```python
from build123d import *

# Parameters (mm, degrees)
SKETCH1_R           = 57.5
SKETCH1_R_2         = 1.75
SKETCH1_R_3         = 26
SKETCH1_R_4         = 2.5
BOSS_EXTRUDE1_DEPTH = 7
SKETCH2_R           = 7
SKETCH2_R_2         = 5
CUT_EXTRUDE1_DEPTH  = 1


with BuildPart() as part:
    # Sketch1 → Boss-Extrude1 (new body)
    with BuildSketch(Plane(origin=(0, 0, 0), x_dir=(1, 0, 0), z_dir=(0, 1, 0))):
        with Locations(Location((0, 0, 0), (0, 0, 270))):
            Circle(SKETCH1_R)
        with Locations(Location((0, 54, 0), (0, 0, 270))):
            Circle(SKETCH1_R_2, mode=Mode.SUBTRACT)
        with Locations(Location((27, 46.765371804, 0), (0, 0, 270))):
            Circle(SKETCH1_R_2, mode=Mode.SUBTRACT)
        with Locations(Location((46.765371804, 27, 0), (0, 0, 270))):
            Circle(SKETCH1_R_2, mode=Mode.SUBTRACT)
        with Locations(Location((54, 0, 0), (0, 0, 270))):
            Circle(SKETCH1_R_2, mode=Mode.SUBTRACT)
        with Locations(Location((46.765371804, -27, 0), (0, 0, 270))):
            Circle(SKETCH1_R_2, mode=Mode.SUBTRACT)
        with Locations(Location((27, -46.765371804, 0), (0, 0, 270))):
            Circle(SKETCH1_R_2, mode=Mode.SUBTRACT)
        with Locations(Location((0, -54, 0), (0, 0, 270))):
            Circle(SKETCH1_R_2, mode=Mode.SUBTRACT)
        with Locations(Location((-27, -46.765371804, 0), (0, 0, 270))):
            Circle(SKETCH1_R_2, mode=Mode.SUBTRACT)
        with Locations(Location((-46.765371804, -27, 0), (0, 0, 270))):
            Circle(SKETCH1_R_2, mode=Mode.SUBTRACT)
        with Locations(Location((-54, 0, 0), (0, 0, 270))):
            Circle(SKETCH1_R_2, mode=Mode.SUBTRACT)
        with Locations(Location((-46.765371804, 27, 0), (0, 0, 270))):
            Circle(SKETCH1_R_2, mode=Mode.SUBTRACT)
        with Locations(Location((-27, 46.765371804, 0), (0, 0, 270))):
            Circle(SKETCH1_R_2, mode=Mode.SUBTRACT)
        with Locations(Location((0, 0, 0), (0, 0, 270))):
            Circle(SKETCH1_R_3, mode=Mode.SUBTRACT)
        with Locations(Location((0, 45, 0), (0, 0, 270))):
            Circle(SKETCH1_R_4, mode=Mode.SUBTRACT)
        with Locations(Location((24.328836786, 37.856408977, 0), (0, 0, 270))):
            Circle(SKETCH1_R_4, mode=Mode.SUBTRACT)
        with Locations(Location((40.933439791, 18.693675585, 0), (0, 0, 270))):
            Circle(SKETCH1_R_4, mode=Mode.SUBTRACT)
        with Locations(Location((44.541964885, -6.404167722, 0), (0, 0, 270))):
            Circle(SKETCH1_R_4, mode=Mode.SUBTRACT)
        with Locations(Location((34.008730846, -29.468733028, 0), (0, 0, 270))):
            Circle(SKETCH1_R_4, mode=Mode.SUBTRACT)
        with Locations(Location((12.677965058, -43.177183813, 0), (0, 0, 270))):
            Circle(SKETCH1_R_4, mode=Mode.SUBTRACT)
        with Locations(Location((-12.677965058, -43.177183813, 0), (0, 0, 270))):
            Circle(SKETCH1_R_4, mode=Mode.SUBTRACT)
        with Locations(Location((-34.008730846, -29.468733028, 0), (0, 0, 270))):
            Circle(SKETCH1_R_4, mode=Mode.SUBTRACT)
        with Locations(Location((-44.541964885, -6.404167722, 0), (0, 0, 270))):
            Circle(SKETCH1_R_4, mode=Mode.SUBTRACT)
        with Locations(Location((-40.933439791, 18.693675585, 0), (0, 0, 270))):
            Circle(SKETCH1_R_4, mode=Mode.SUBTRACT)
        with Locations(Location((-24.328836786, 37.856408977, 0), (0, 0, 270))):
            Circle(SKETCH1_R_4, mode=Mode.SUBTRACT)
    extrude(amount=BOSS_EXTRUDE1_DEPTH)

    # Sketch2 → Cut-Extrude1 (cut)
    # profile 1 of 11: a face of its own
    with BuildSketch(Plane(origin=(0, 7, 0), x_dir=(1, 0, 0), z_dir=(0, 1, 0))):
        with Locations(Location((0, 45, 0), (0, 0, 270))):
            Circle(SKETCH2_R)
        with Locations(Location((0, 45, 0), (0, 0, 270))):
            Circle(SKETCH2_R_2, mode=Mode.SUBTRACT)
    # profile 2 of 11: a face of its own
    with BuildSketch(Plane(origin=(0, 7, 0), x_dir=(1, 0, 0), z_dir=(0, 1, 0))):
        with Locations(Location((24.328836786, 37.856408977, 0), (0, 0, 270))):
            Circle(SKETCH2_R)
        with Locations(Location((24.328836786, 37.856408977, 0), (0, 0, 270))):
            Circle(SKETCH2_R_2, mode=Mode.SUBTRACT)
    # profile 3 of 11: a face of its own
    with BuildSketch(Plane(origin=(0, 7, 0), x_dir=(1, 0, 0), z_dir=(0, 1, 0))):
        with Locations(Location((40.933439791, 18.693675585, 0), (0, 0, 270))):
            Circle(SKETCH2_R)
        with Locations(Location((40.933439791, 18.693675585, 0), (0, 0, 270))):
            Circle(SKETCH2_R_2, mode=Mode.SUBTRACT)
    # profile 4 of 11: a face of its own
    with BuildSketch(Plane(origin=(0, 7, 0), x_dir=(1, 0, 0), z_dir=(0, 1, 0))):
        with Locations(Location((44.541964885, -6.404167722, 0), (0, 0, 270))):
            Circle(SKETCH2_R)
        with Locations(Location((44.541964885, -6.404167722, 0), (0, 0, 270))):
            Circle(SKETCH2_R_2, mode=Mode.SUBTRACT)
    # profile 5 of 11: a face of its own
    with BuildSketch(Plane(origin=(0, 7, 0), x_dir=(1, 0, 0), z_dir=(0, 1, 0))):
        with Locations(Location((34.008730846, -29.468733028, 0), (0, 0, 270))):
            Circle(SKETCH2_R)
        with Locations(Location((34.008730846, -29.468733028, 0), (0, 0, 270))):
            Circle(SKETCH2_R_2, mode=Mode.SUBTRACT)
    # profile 6 of 11: a face of its own
    with BuildSketch(Plane(origin=(0, 7, 0), x_dir=(1, 0, 0), z_dir=(0, 1, 0))):
        with Locations(Location((12.677965058, -43.177183813, 0), (0, 0, 270))):
            Circle(SKETCH2_R)
        with Locations(Location((12.677965058, -43.177183813, 0), (0, 0, 270))):
            Circle(SKETCH2_R_2, mode=Mode.SUBTRACT)
    # profile 7 of 11: a face of its own
    with BuildSketch(Plane(origin=(0, 7, 0), x_dir=(1, 0, 0), z_dir=(0, 1, 0))):
        with Locations(Location((-12.677965058, -43.177183813, 0), (0, 0, 270))):
            Circle(SKETCH2_R)
        with Locations(Location((-12.677965058, -43.177183813, 0), (0, 0, 270))):
            Circle(SKETCH2_R_2, mode=Mode.SUBTRACT)
    # profile 8 of 11: a face of its own
    with BuildSketch(Plane(origin=(0, 7, 0), x_dir=(1, 0, 0), z_dir=(0, 1, 0))):
        with Locations(Location((-34.008730846, -29.468733028, 0), (0, 0, 270))):
            Circle(SKETCH2_R)
        with Locations(Location((-34.008730846, -29.468733028, 0), (0, 0, 270))):
            Circle(SKETCH2_R_2, mode=Mode.SUBTRACT)
    # profile 9 of 11: a face of its own
    with BuildSketch(Plane(origin=(0, 7, 0), x_dir=(1, 0, 0), z_dir=(0, 1, 0))):
        with Locations(Location((-44.541964885, -6.404167722, 0), (0, 0, 270))):
            Circle(SKETCH2_R)
        with Locations(Location((-44.541964885, -6.404167722, 0), (0, 0, 270))):
            Circle(SKETCH2_R_2, mode=Mode.SUBTRACT)
    # profile 10 of 11: a face of its own
    with BuildSketch(Plane(origin=(0, 7, 0), x_dir=(1, 0, 0), z_dir=(0, 1, 0))):
        with Locations(Location((-40.933439791, 18.693675585, 0), (0, 0, 270))):
            Circle(SKETCH2_R)
        with Locations(Location((-40.933439791, 18.693675585, 0), (0, 0, 270))):
            Circle(SKETCH2_R_2, mode=Mode.SUBTRACT)
    # profile 11 of 11: a face of its own
    with BuildSketch(Plane(origin=(0, 7, 0), x_dir=(1, 0, 0), z_dir=(0, 1, 0))):
        with Locations(Location((-24.328836786, 37.856408977, 0), (0, 0, 270))):
            Circle(SKETCH2_R)
        with Locations(Location((-24.328836786, 37.856408977, 0), (0, 0, 270))):
            Circle(SKETCH2_R_2, mode=Mode.SUBTRACT)
    extrude(amount=-CUT_EXTRUDE1_DEPTH, mode=Mode.SUBTRACT)


solid = part.part
```
Read the model definition and answer for the solid it produces. Units are mm, in the model's axes. A direction names the side the tool comes from. Give positions to 0.01 mm unless a question says otherwise; leave off trailing zeros. Order: outer loops, then holes, each group sorted by start corner. A loop starts at its lowest first (then second) coordinate and runs counter-clockwise, first axis right, second up.
(1) Given pin 1 (2 mm diameter, centred on y = 1.5, z = 10, fed in from -X); pin 2 (1.5 mm diameter, centred on y = 4.5, z = 19.5, fed in from +X); pin 3 (3 mm diameter, centred on x = -32.5, y = 1, fed in from +Z), each flat-ended and moving along its own axis, determine where each tip first touches the part or whether it passes through.
(2) Find section B-B (z = 54). Give the vertices of the cut face in (x, y).
(3) Find section A-A (x = 0). Give the vertices of the cut face in (y, z), plus the area to 3 significant figures.
(4) For faces 3 (the cylindrical face through (-38.825, 3.451, -17.35)), 4 (the cylindrical face through (-37.6, 6.5, 5.5)), determine the directions among +Z, -Z, +X, -X, +Y, -Y from which every point of the face is accessible in a straight line to the end or side of a thin tool.
(5) Find section D-D (x = 54). Give the vertices of the cut face in (y, z).
(6) Find section C-C (y = 1.5). Give the number of separate pieces and of enclosed holes in the cut face, plus the area to 3 significant figures.
(7) Straight lines are drawn through the part: L1, parallel to Z at x = 20, y = 6.25; L2, parallel to X at y = 4.75, z = -37.5; L3, parallel to Z at x = 23.5, y = 1.25. For each, find the intervals that lie inside material, in ascending order.
(8) For a pull along Z with two mould halves and no side action, classify faces 1 (the cylindrical face through (-28.6, 6.5, -43.4)), 2 (the flat face through (-43, 7, -17)) as released by +Z, released by -Z, zero draft, split by the parting line, or undercut.
Result sheet:
1. pin 1: stops at x = -56.79
1. pin 2: stops at x = 54.36
1. pin 3: stops at z = 48.43
2. outline: (-19.75, 0) - (-1.75, 0) - (-1.75, 7) - (-19.75, 7) - close; (1.75, 0) - (19.75, 0) - (19.75, 7) - (1.75, 7) - close
3. outline: (0, -57.5) - (7, -57.5) - (7, -55.75) - (0, -55.75) - close; (0, -52.25) - (7, -52.25) - (7, -52) - (6, -52) - (6, -50) - (7, -50) - (7, -47.5) - (0, -47.5) - close; (0, -42.5) - (7, -42.5) - (7, -40) - (6, -40) - (6, -38) - (7, -38) - (7, -26) - (0, -26) - close; (0, 26) - (7, 26) - (7, 52.25) - (0, 52.25) - close; (0, 55.75) - (7, 55.75) - (7, 57.5) - (0, 57.5) - close
3. area: 353 mm2
4. face 3: +Y, -Y
4. face 4: +Y
5. outline: (0, -19.75) - (7, -19.75) - (7, -1.75) - (0, -1.75) - close; (0, 1.75) - (7, 1.75) - (7, 19.75) - (0, 19.75) - close
6. separate pieces: 1
6. enclosed holes: 24
6. area: 7,930 mm2
7. L1: z = -53.91 to -43.36, -40.36 to -35.35, -32.36 to -16.61, 16.61 to 53.91
7. L2: x = -43.59 to -26.8, -21.85 to 21.85, 26.8 to 43.59
7. L3: z = -52.48 to -40.22, -35.5 to -11.12, 11.12 to 52.48
8. face 1: undercut
8. face 2: zero draft
